```python
from build123d import *

# Parameters (mm, degrees)
SKETCH_W            = 152.4
SKETCH_H            = 63.5
PAD_DEPTH           = 25.4
SKETCH001_W         = 146.05
SKETCH001_H         = 56.642
PAD001_DEPTH        = 5.08
SKETCH002_W         = 142.367
SKETCH002_H         = 53.975
POCKET_DEPTH        = 28.575
FILLET_R            = 1.27
CHAMFER_SIZE        = 12.7
SKETCH003_R         = 1.8669
HOLE_DEPTH          = 19.05
HOLE_TIPS_R         = 1.8669
SKETCH004_R         = 14.986
POCKET001_DEPTH     = 12.7
SKETCH006_R         = 18.288
POCKET003_DEPTH     = 5.0038
SKETCH007_R         = 4.064
PAD002_DEPTH        = 7.8994
SKETCH008_R         = 1.524
HOLE001_DEPTH       = 8.89
HOLE001_TIPS_R      = 1.524
SKETCH010_W         = 0.958809
SKETCH010_H         = 53.975
PAD003_DEPTH        = 7.8994
SKETCH011_W         = 6.35
SKETCH011_H         = 6.985
PAD004_DEPTH        = 27.94
SKETCH012_R         = 1.8669
HOLE002_DEPTH       = 19.05
HOLE002_TIPS_R      = 1.8669
HOLE003_D           = 2.9
HOLE003_DEPTH       = 24.9936
HOLE003_CSINK_D     = 6.1
HOLE003_CSINK_ANGLE = 90
HOLE003_TIPS_R      = 1.45
SKETCH015_R         = 4.445
PAD005_DEPTH        = 3.175
SKETCH016_R         = 2.667
HOLE004_DEPTH       = 12.7
HOLE004_TIPS_R      = 2.667
SKETCH017_R         = 4.445
PAD006_DEPTH        = 3.175
SKETCH018_R         = 2.667
HOLE005_DEPTH       = 12.7
HOLE005_TIPS_R      = 2.667
SKETCH009_W         = 65.405
SKETCH009_H         = 27.94
PAD007_DEPTH        = 3.048
SKETCH005_W         = 60.452
SKETCH005_H         = 19.6088
POCKET004_DEPTH     = 10.16
SKETCH019_W         = 63.5
SKETCH019_H         = 25.4
POCKET005_DEPTH     = 3.175


with BuildPart() as part:
    # Sketch → Pad (new body)
    with BuildSketch(Plane.XY):
        Rectangle(SKETCH_W, SKETCH_H)
    extrude(amount=PAD_DEPTH)

    # Sketch001 (on Face6 of Pad) → Pad001 (join)
    with BuildSketch(Plane.XY.offset(25.4)):
        Rectangle(SKETCH001_W, SKETCH001_H)
    extrude(amount=PAD001_DEPTH)

    # Sketch002 (on Face11 of Pad001) → Pocket (cut)
    with BuildSketch(Plane.XY.offset(30.48)):
        Rectangle(SKETCH002_W, SKETCH002_H)
    extrude(amount=-POCKET_DEPTH, mode=Mode.SUBTRACT)

    # Fillet
    fillet_edges = [part.edges().sort_by_distance(p)[0] for p in [
        (0, 31.75, 0),
        (-76.2, 0, 0),
        (0, -31.75, 0),
        (76.2, 0, 0),
        (-76.2, 31.75, 12.7),
        (76.2, 31.75, 12.7),
        (76.2, -31.75, 12.7),
        (-76.2, -31.75, 12.7),
    ]]
    fillet(fillet_edges, radius=FILLET_R)

    # Chamfer
    chamfer_edges = [part.edges().sort_by_distance(p)[0] for p in [
        (-71.1835, 26.9875, 16.1925),
        (-71.1835, -26.9875, 16.1925),
    ]]
    chamfer(chamfer_edges, length=CHAMFER_SIZE)

    # Sketch003 (on Face1 of Chamfer) → Hole (cut)
    with BuildSketch(Plane.XY.offset(30.48)):
        with Locations((-68.58, 24.13)):
            Circle(SKETCH003_R)
        with Locations((-68.58, -24.13)):
            Circle(SKETCH003_R)
    extrude(amount=-HOLE_DEPTH, mode=Mode.SUBTRACT)

    # Hole tips → Hole tip 1 section 0
    with BuildSketch(Plane.XY.offset(11.43), mode=Mode.PRIVATE) as hole_tip_1_s0:
        with Locations((-68.58, 24.13)):
            Circle(HOLE_TIPS_R)
    loft([hole_tip_1_s0.sketch, Vertex(-68.58, 24.13, 10.308253)], mode=Mode.SUBTRACT)

    # Hole tips → Hole tip 2 section 0
    with BuildSketch(Plane.XY.offset(11.43), mode=Mode.PRIVATE) as hole_tip_2_s0:
        with Locations((-68.58, -24.13)):
            Circle(HOLE_TIPS_R)
    loft([hole_tip_2_s0.sketch, Vertex(-68.58, -24.13, 10.308253)], mode=Mode.SUBTRACT)

    # Sketch004 (on Face25 of Hole) → Pocket001 (cut)
    with BuildSketch(Plane.YZ.offset(76.2)):
        with Locations((3.175, 25.4)):
            Circle(SKETCH004_R)
    extrude(amount=-POCKET001_DEPTH, mode=Mode.SUBTRACT)

    # Sketch006 → Pocket003 (cut)
    with BuildSketch(Plane(origin=(0, 0, 0), x_dir=(1, 0, 0), z_dir=(0, 0, -1))):
        with Locations((-47.625, 0)):
            Circle(SKETCH006_R)
    extrude(amount=-POCKET003_DEPTH, mode=Mode.SUBTRACT)

    # Sketch007 (on Face18 of Pocket003) → Pad002 (join)
    with BuildSketch(Plane.XY.offset(1.905)):
        with Locations((-63.754, 16.129)):
            Circle(SKETCH007_R)
        with Locations((-31.496, 16.129)):
            Circle(SKETCH007_R)
        with Locations((-31.496, -16.129)):
            Circle(SKETCH007_R)
        with Locations((-63.754, -16.129)):
            Circle(SKETCH007_R)
    extrude(amount=PAD002_DEPTH)

    # Sketch008 (on Face19 of Pad002) → Hole001 (cut)
    with BuildSketch(Plane.XY.offset(9.8044)):
        with Locations((-63.754, 16.129)):
            Circle(SKETCH008_R)
        with Locations((-31.496, 16.129)):
            Circle(SKETCH008_R)
        with Locations((-31.496, -16.129)):
            Circle(SKETCH008_R)
        with Locations((-63.754, -16.129)):
            Circle(SKETCH008_R)
    extrude(amount=-HOLE001_DEPTH, mode=Mode.SUBTRACT)

    # Hole001 tips → Hole001 tip 1 section 0
    with BuildSketch(Plane.XY.offset(0.9144), mode=Mode.PRIVATE) as hole001_tip_1_s0:
        with Locations((-63.754, 16.129)):
            Circle(HOLE001_TIPS_R)
    loft([hole001_tip_1_s0.sketch, Vertex(-63.754, 16.129, -0.001312)], mode=Mode.SUBTRACT)

    # Hole001 tips → Hole001 tip 2 section 0
    with BuildSketch(Plane.XY.offset(0.9144), mode=Mode.PRIVATE) as hole001_tip_2_s0:
        with Locations((-31.496, 16.129)):
            Circle(HOLE001_TIPS_R)
    loft([hole001_tip_2_s0.sketch, Vertex(-31.496, 16.129, -0.001312)], mode=Mode.SUBTRACT)

    # Hole001 tips → Hole001 tip 3 section 0
    with BuildSketch(Plane.XY.offset(0.9144), mode=Mode.PRIVATE) as hole001_tip_3_s0:
        with Locations((-31.496, -16.129)):
            Circle(HOLE001_TIPS_R)
    loft([hole001_tip_3_s0.sketch, Vertex(-31.496, -16.129, -0.001312)], mode=Mode.SUBTRACT)

    # Hole001 tips → Hole001 tip 4 section 0
    with BuildSketch(Plane.XY.offset(0.9144), mode=Mode.PRIVATE) as hole001_tip_4_s0:
        with Locations((-63.754, -16.129)):
            Circle(HOLE001_TIPS_R)
    loft([hole001_tip_4_s0.sketch, Vertex(-63.754, -16.129, -0.001312)], mode=Mode.SUBTRACT)

    # Sketch010 → Pad003 (join)
    with BuildSketch(Plane.XY.offset(1.905)):
        with Locations((-27.854217, 0)):
            Rectangle(SKETCH010_W, SKETCH010_H)
    extrude(amount=PAD003_DEPTH)

    # Sketch011 (on Face18 of Pad003) → Pad004 (join)
    with BuildSketch(Plane.XY.offset(1.905)):
        with Locations((47.625, 23.495)):
            Rectangle(SKETCH011_W, SKETCH011_H)
        with Locations((47.625, -23.495)):
            Rectangle(SKETCH011_W, SKETCH011_H)
    extrude(amount=PAD004_DEPTH)

    # Sketch012 (on Face24 of Pad004) → Hole002 (cut)
    with BuildSketch(Plane.XY.offset(29.845)):
        with Locations((47.625, 23.368)):
            Circle(SKETCH012_R)
        with Locations((47.625, -23.368)):
            Circle(SKETCH012_R)
    extrude(amount=-HOLE002_DEPTH, mode=Mode.SUBTRACT)

    # Hole002 tips → Hole002 tip 1 section 0
    with BuildSketch(Plane.XY.offset(10.795), mode=Mode.PRIVATE) as hole002_tip_1_s0:
        with Locations((47.625, 23.368)):
            Circle(HOLE002_TIPS_R)
    loft([hole002_tip_1_s0.sketch, Vertex(47.625, 23.368, 9.673253)], mode=Mode.SUBTRACT)

    # Hole002 tips → Hole002 tip 2 section 0
    with BuildSketch(Plane.XY.offset(10.795), mode=Mode.PRIVATE) as hole002_tip_2_s0:
        with Locations((47.625, -23.368)):
            Circle(HOLE002_TIPS_R)
    loft([hole002_tip_2_s0.sketch, Vertex(47.625, -23.368, 9.673253)], mode=Mode.SUBTRACT)

    # Hole003
    with Locations(Plane.YZ.offset(76.2)):
        with Locations((-11.811, 10.3378), (18.3134, 10.3378)):
            CounterSinkHole(HOLE003_D / 2, HOLE003_CSINK_D / 2, depth=HOLE003_DEPTH, counter_sink_angle=HOLE003_CSINK_ANGLE)

    # Hole003 tips → Hole003 tip 1 section 0
    with BuildSketch(Plane.YZ.offset(51.2064), mode=Mode.PRIVATE) as hole003_tip_1_s0:
        with Locations((-11.811, 10.3378)):
            Circle(HOLE003_TIPS_R)
    loft([hole003_tip_1_s0.sketch, Vertex(50.335152, -11.811, 10.3378)], mode=Mode.SUBTRACT)

    # Hole003 tips → Hole003 tip 2 section 0
    with BuildSketch(Plane.YZ.offset(51.2064), mode=Mode.PRIVATE) as hole003_tip_2_s0:
        with Locations((18.3134, 10.3378)):
            Circle(HOLE003_TIPS_R)
    loft([hole003_tip_2_s0.sketch, Vertex(50.335152, 18.3134, 10.3378)], mode=Mode.SUBTRACT)

    # Sketch015 → Pad005 (join)
    with BuildSketch(Plane(origin=(0, -26.9875, 0), x_dir=(-1, 0, 0), z_dir=(0, 1, 0))):
        with Locations((-41.177467, 15.875)):
            Circle(SKETCH015_R)
        with Locations((41.342368, 15.875)):
            Circle(SKETCH015_R)
    extrude(amount=PAD005_DEPTH)

    # Sketch016 (on Face43 of Pad005) → Hole004 (cut)
    with BuildSketch(Plane.XZ.offset(31.75)):
        with Locations((-41.275, 15.875)):
            Circle(SKETCH016_R)
        with Locations((41.275, 15.875)):
            Circle(SKETCH016_R)
    extrude(amount=-HOLE004_DEPTH, mode=Mode.SUBTRACT)

    # Hole004 tips → Hole004 tip 1 section 0
    with BuildSketch(Plane.XZ.offset(19.05), mode=Mode.PRIVATE) as hole004_tip_1_s0:
        with Locations((-41.275, 15.875)):
            Circle(HOLE004_TIPS_R)
    loft([hole004_tip_1_s0.sketch, Vertex(-41.275, -17.447505, 15.875)], mode=Mode.SUBTRACT)

    # Hole004 tips → Hole004 tip 2 section 0
    with BuildSketch(Plane.XZ.offset(19.05), mode=Mode.PRIVATE) as hole004_tip_2_s0:
        with Locations((41.275, 15.875)):
            Circle(HOLE004_TIPS_R)
    loft([hole004_tip_2_s0.sketch, Vertex(41.275, -17.447505, 15.875)], mode=Mode.SUBTRACT)

    # Sketch017 (on Face6 of Hole004) → Pad006 (join)
    with BuildSketch(Plane.XZ.offset(-26.9875)):
        with Locations((-41.3385, 15.875)):
            Circle(SKETCH017_R)
        with Locations((41.2115, 15.875)):
            Circle(SKETCH017_R)
    extrude(amount=PAD006_DEPTH)

    # Sketch018 (on Face43 of Pad006) → Hole005 (cut)
    with BuildSketch(Plane(origin=(0, 31.75, 0), x_dir=(-1, 0, 0), z_dir=(0, 1, 0))):
        with Locations((-41.275, 15.875)):
            Circle(SKETCH018_R)
        with Locations((41.275, 15.875)):
            Circle(SKETCH018_R)
    extrude(amount=-HOLE005_DEPTH, mode=Mode.SUBTRACT)

    # Hole005 tips → Hole005 tip 1 section 0
    with BuildSketch(Plane(origin=(0, 19.05, 0), x_dir=(-1, 0, 0), z_dir=(0, 1, 0)), mode=Mode.PRIVATE) as hole005_tip_1_s0:
        with Locations((-41.275, 15.875)):
            Circle(HOLE005_TIPS_R)
    loft([hole005_tip_1_s0.sketch, Vertex(41.275, 17.447505, 15.875)], mode=Mode.SUBTRACT)

    # Hole005 tips → Hole005 tip 2 section 0
    with BuildSketch(Plane(origin=(0, 19.05, 0), x_dir=(-1, 0, 0), z_dir=(0, 1, 0)), mode=Mode.PRIVATE) as hole005_tip_2_s0:
        with Locations((41.275, 15.875)):
            Circle(HOLE005_TIPS_R)
    loft([hole005_tip_2_s0.sketch, Vertex(-41.275, 17.447505, 15.875)], mode=Mode.SUBTRACT)

    # Sketch009 (on Face18 of Hole001) → Pad007 (join)
    with BuildSketch(Plane.XY.offset(1.905)):
        with Locations((7.9375, 0.0254)):
            Rectangle(SKETCH009_W, SKETCH009_H)
    extrude(amount=PAD007_DEPTH)

    # Sketch005 (on Face35 of Pocket001) → Pocket004 (cut)
    with BuildSketch(Plane(origin=(0, 0, 0), x_dir=(1, 0, 0), z_dir=(0, 0, -1))):
        with Locations((7.874, 0)):
            Rectangle(SKETCH005_W, SKETCH005_H)
    extrude(amount=-POCKET004_DEPTH, mode=Mode.SUBTRACT)

    # Sketch019 (on Face84 of Pocket004) → Pocket005 (cut)
    with BuildSketch(Plane.XY.offset(4.953)):
        with Locations((7.956801, -0.2794)):
            Rectangle(SKETCH019_W, SKETCH019_H)
    extrude(amount=-POCKET005_DEPTH, mode=Mode.SUBTRACT)


solid = part.part
```
The model under review builds one solid part; all positions refer to its coordinate system, in mm. A direction names the side the tool comes from. Round coordinates to 2 decimals unless told otherwise and drop trailing zeros. Use CSV: the item, a comma, the result in double quotes.
Q1. To check wall thickness, follow probe 1 along Y at (x, z) = (-51.5, 13); probe 2 along Y at (x, z) = (-70, 27.5); probe 3 along Y at (x, z) = (47.5, 27.5). State the ranges of each line that lie inside material, in increasing order. Write a range as [from, to].
Checks:
probe 1,"[-31.75, -26.99], [26.99, 31.75]"
probe 2,"[-28.32, -25.34], [-22.92, -15.47], [15.47, 22.92], [25.34, 28.32]"
probe 3,"[-28.32, -25.23], [-21.51, -20], [20, 21.51], [25.23, 28.32]"
Q2. For pin 1 Ø6 at (x, y) = (-56.5, -18) entering from +Z (3 decimals); pin 2 Ø7 at (x, z) = (41.275, 15.875) entering from -Y; pin 3 Ø1.9 at (x, y) = (48.5, 24.5) entering from +Z (3 decimals); pin 4 Ø3 at (x, y) = (-37.5, 23) entering from +Z, all flat-tipped, find the tip position at first contact; note any pin that passes through.
Checks:
pin 1,"z = 1.905"
pin 2,"y = -31.75"
pin 3,"z = 29.845"
pin 4,"z = 19.5"
Q3. Consider section B-B (y = 0). State how many separate pieces and enclosed holes the cut face has, then the cut area to 3 significant figures.
Checks:
separate pieces,"3"
enclosed holes,"0"
area,"289 mm²"
Q4. Mouldability with a two-part tool opening along Y and no side actions: class faces 1 (the flat face through (-16.6, 27.4, 30.48)), 2 (the flat face through (-1, 28.321, 28)), 3 (the flat face through (-28.334, 0, 6)) as released by +Y, released by -Y, zero draft, split by the parting line, or undercut.
Checks:
face 1,"zero draft"
face 2,"released by +Y"
face 3,"undercut"
Q5. For faces 4 (the cylindrical face through (-65.277, -16.062, 5.422)), 5 (the cylindrical face through (36.77, 25.42, 16.02)), 6 (the flat face through (-1, 31.75, 13)), list the 3-axis set-ups (+Z, -Z, +X, -X, +Y, -Y) from which the entire face can be reached by the end or side of a thin tool; tool diameter is ignored.
Checks:
face 4,"+Z"
face 5,"none"
face 6,"+Z, -Z, +X, -X, +Y"
